from build123d import *

# Parameters (mm, degrees)
F0_R     = 25.687791
F0_R_2   = 17.294442
F1_DEPTH = 10.922
F2_DEPTH = 39.37
F3_R     = 8.773481
F4_DEPTH = 19.812


with BuildPart() as f1:
    # F0 (on Top) → F1 (new body)
    with BuildSketch(Plane.XY):
        Circle(F0_R)
        Circle(F0_R_2, mode=Mode.SUBTRACT)
        Circle(F0_R_2)
    extrude(amount=F1_DEPTH)

    # F0 (on Top) → F2 (join)
    with BuildSketch(Plane.XY):
        Circle(F0_R_2)
    extrude(amount=F2_DEPTH)

    # F3 (on face) → F4 (cut)
    with BuildSketch(Plane.XY.offset(39.37)):
        Circle(F3_R)
    extrude(amount=-F4_DEPTH, mode=Mode.SUBTRACT)


solid = f1.part
Could you check a few things on this model? Use its own coordinates, in mm. A direction names the side the tool comes from. Coordinates: 2 decimals unless noted, no trailing zeros. Order: outer loops, then holes, each group sorted by start corner. A loop starts at its lowest first (then second) coordinate and runs counter-clockwise, first axis right, second up. Notation, with made-up numbers: (-27.5, 46) -> (-15.5, 46) arc R25 cw to (-15.5, 58) -> close; hole circle Ø3 at (54, 72). An arc over 180 degrees is marked (long way). One line per item, written item: value. Start each with the question number.
1) Imagine slicing it at C-C on z = 16.5. List the corners of the cut face in (x, y) for me, plus the area to 3 significant figures.
2) We'd pull the mould along Y, two halves only. Please class faces 1 (the cylindrical face through (16.496, 5.195, 24.947)), 2 (the flat face through (17, -5, 10.922)), 3 (the flat face through (0, 0, 19.558)): +Y half, -Y half, draft (parallel to the pull), parting line (faces both ways), or undercut.
3) Imagine slicing it at A-A on x = 0. List the corners of the cut face in (y, z) for me, plus the area to 3 significant figures.
4) I'm going to push flat-ended pins straight in: pin 1 (6 mm diameter, centred on x = 4, z = 12, fed in from -Y); pin 2 (6 mm diameter, centred on x = 2, z = 32.5, fed in from +Y); pin 3 (4 mm diameter, centred on y = 10.5, z = 5, fed in from +X). Where does each tip first touch, or does it pass through?
5) If I drill on L1, parallel to Y at x = 0, z = 31; L2, parallel to Z at x = -1, y = -8; L3, parallel to Y at x = 5.5, z = 25.5, over which ranges is the centre line in solid material (lowest first)? Write a range as [from, to].
6) Imagine slicing it at D-D on z = 28.5. List the corners of the cut face in (x, y) for me.
7) Which directions (+Z, -Z, +X, -X, +Y, -Y) give clear straight access to the entire face, cutting with the end or side of a thin tool? Please do faces 4 (the cylindrical face through (-6.96, -5.34, 29.6)), 5 (the cylindrical face through (-20.385, -15.631, 5.385)).
Answer list:
1. outline: circle Ø34.59 at (0, 0)
1. area: 940 mm2
2. face 1: parting line
2. face 2: draft
2. face 3: undercut
3. outline: (-25.69, 0) -> (25.69, 0) -> (25.69, 10.92) -> (17.29, 10.92) -> (17.29, 39.37) -> (8.77, 39.37) -> (8.77, 19.56) -> (-8.77, 19.56) -> (-8.77, 39.37) -> (-17.29, 39.37) -> (-17.29, 10.92) -> (-25.69, 10.92) -> close
3. area: 1,200 mm2
4. pin 1: stops at y = -25.66
4. pin 2: stops at y = 17.29
4. pin 3: stops at x = 24.24
5. L1: y = [-17.29, -8.77], [8.77, 17.29]
5. L2: z = [0, 19.56]
5. L3: y = [-16.4, -6.84], [6.84, 16.4]
6. outline: circle Ø34.59 at (0, 0); hole circle Ø17.55 at (0, 0)
7. face 4: +Z
7. face 5: +Z, -Z
